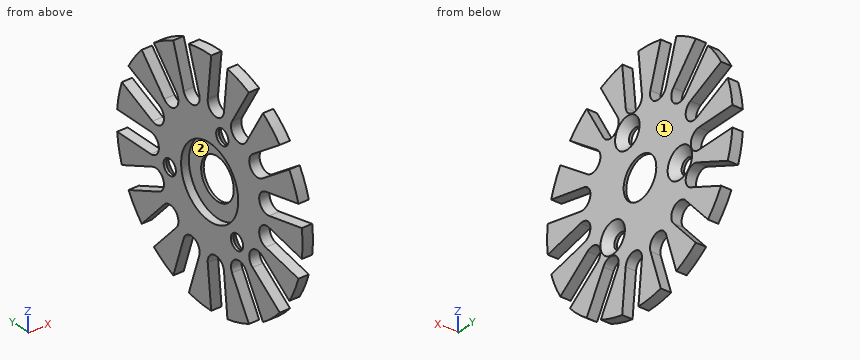
from build123d import *

# Parameters (mm, degrees)
SKETCH1_R                    = 22.75
BOSS_EXTRUDE1_DEPTH          = 2
CUT_EXTRUDE2_REACH           = 4
SKETCH3_R                    = 4
SKETCH2_R                    = 1.5
CUT_EXTRUDE1_DEPTH           = 2
CHAMFER1_SIZE                = 1.5
CIRPATTERN1_COUNT            = 3
CHAMFER1_OF_CIRPATTERN1_SIZE = 1.5
CUT_EXTRUDE3_DEPTH           = 2
CIRPATTERN2_COUNT            = 15
SKETCH5_R                    = 7
CUT_EXTRUDE4_DEPTH           = 1.5


with BuildPart() as part:
    # Sketch1 → Boss-Extrude1 (new body)
    with BuildSketch(Plane(origin=(0, 0, 0), x_dir=(0, 0, -1), z_dir=(1, 0, 0))):
        Circle(SKETCH1_R)
    extrude(amount=BOSS_EXTRUDE1_DEPTH)

    # Sketch3 → Cut-Extrude2 (cut, up to next)
    with BuildSketch(Plane(origin=(2, 0, 0), x_dir=(0, 0, -1), z_dir=(1, 0, 0)), mode=Mode.PRIVATE) as cut_extrude2_sk1:
        Circle(SKETCH3_R)
    cut_extrude2_tool1 = extrude(cut_extrude2_sk1.sketch, amount=-CUT_EXTRUDE2_REACH, mode=Mode.PRIVATE) & part.part
    add(cut_extrude2_tool1.solids().sort_by_distance((2, 0, 0))[0], mode=Mode.SUBTRACT)

    # Sketch2 → Cut-Extrude1 (cut)
    with BuildSketch(Plane(origin=(2, 0, 0), x_dir=(0, 0, -1), z_dir=(1, 0, 0))):
        with Locations((2.079116908, 9.781476007)):
            Circle(SKETCH2_R)
    cut_extrude1 = extrude(amount=-CUT_EXTRUDE1_DEPTH, mode=Mode.SUBTRACT)

    # Chamfer1
    chamfer1_edges = [part.edges().sort_by_distance(p)[0] for p in [
        (2, 9.781476007, -0.579116908),
    ]]
    chamfer(chamfer1_edges, length=CHAMFER1_SIZE)

    # CirPattern1: Cut-Extrude1 ×3 about axis
    cirpattern1_axis = Axis((0, 0, 0), (1, 0, 0))
    for i in range(1, CIRPATTERN1_COUNT):
        add(cut_extrude1.rotate(cirpattern1_axis, i * 360 / CIRPATTERN1_COUNT), mode=Mode.SUBTRACT)

    # Chamfer1 of CirPattern1
    chamfer1_of_cirpattern1_edges = [part.edges().sort_by_distance(p)[0] for p in [
        (2, -4.389208049, 8.760565163),
        (2, -5.392267958, -8.181448255),
    ]]
    chamfer(chamfer1_of_cirpattern1_edges, length=CHAMFER1_OF_CIRPATTERN1_SIZE)

    # Sketch4 → Cut-Extrude3 (cut)
    with BuildSketch(Plane(origin=(2, 0, 0), x_dir=(0, 0, -1), z_dir=(1, 0, 0))):
        with BuildLine():
            Line((-2, 22.75), (-2, 14.45))
            ThreePointArc((-2, 14.45), (0, 12.45), (2, 14.45))
            Line((2, 14.45), (2, 22.75))
            Line((2, 22.75), (-2, 22.75))
        make_face()
    cut_extrude3 = extrude(amount=-CUT_EXTRUDE3_DEPTH, mode=Mode.SUBTRACT)

    # CirPattern2: Cut-Extrude3 ×15 about axis
    cirpattern2_axis = Axis((0, 0, 0), (1, 0, 0))
    for i in range(1, CIRPATTERN2_COUNT):
        add(cut_extrude3.rotate(cirpattern2_axis, i * 360 / CIRPATTERN2_COUNT), mode=Mode.SUBTRACT)

    # Sketch5 → Cut-Extrude4 (cut)
    with BuildSketch(Plane.ZY):
        Circle(SKETCH5_R)
    extrude(amount=-CUT_EXTRUDE4_DEPTH, mode=Mode.SUBTRACT)


solid = part.part
Input: part model. Units: mm. Frame: model coordinates. Face numbers are marked on the shaded views. Coordinates: 2 decimals unless noted, no trailing zeros. Order: outer loops, then holes, each group sorted by start corner. A loop starts at its lowest first (then second) coordinate and runs counter-clockwise, first axis right, second up. Notation, with made-up numbers: M -7.5,38.25 L 34.5,38.25 A20 cw 34.5,49.25 Z; hole C 53.5,-2.75 d7. An arc over 180 degrees is marked long. Answer as CSV lines item,"result".
1. Section A-A (y = 16). Return the cut outline in (x, z), then the cut area to 3 significant figures.
Reported:
outline,"M 0,-14.78 L 2,-14.78 L 2,-9.31 L 0,-9.31 Z; M 0,-4.93 L 2,-4.93 L 2,-2 L 0,-2 Z; M 0,2 L 2,2 L 2,4.93 L 0,4.93 Z; M 0,9.31 L 2,9.31 L 2,14.78 L 0,14.78 Z"
area,"33.6 mm2"
2. Pull-direction query (Z, two-part tool) for the marked faces 1 and 2; classes: released by +Z, released by -Z, zero draft, split by the parting line, or undercut.
Reported:
face 1,"zero draft"
face 2,"undercut"
3. Section B-B (x = 0.9). State how many separate pieces and enclosed holes the cut face has, then the cut area to 3 significant figures.
Reported:
separate pieces,"1"
enclosed holes,"4"
area,"848 mm2"
4. Material intervals for line 1 (Z direction, x = 1.35, y = -13); line 2 (Z direction, x = 1.6, y = -13.5); line 3 (Y direction, x = 0.45, z = 18), sorted ascending. Write a range as from..to.
Reported:
line 1,"-18.52..-11.92, -6.97..-4.65, -1.36..1.36, 4.65..6.97, 11.92..18.52"
line 2,"-18.31..-12.28, -7.34..-4.9, -1.11..1.11, 4.9..7.34, 12.28..18.31"
line 3,"-13.91..-12.7, -8.08..-3.9, 0.12..3.75, 7.95..13.52"
5. First-contact query: P1, Ø2.5, axis at y = -3.09, z = 9.51, coming from the +X side; P2, Ø16, axis at y = 0, z = 0, coming from the +X side; P3, Ø1, axis at x = 0.5, z = 6, coming from the +Y side; P4, Ø4, axis at y = 2.5, z = 0, coming from the -X side. Flat tips, straight axial feed; report the tip coordinate or a pass-through.
Reported:
P1,"through"
P2,"x = 2"
P3,"y = 22.08"
P4,"x = 1.5"
